Check sheet for the modelled part. Datum: model origin and axes. Units: mm. A direction names the side the tool comes from. Coordinates: 2 decimals unless noted, no trailing zeros. Loops run counter-clockwise (first coordinate to the right, second up) from the corner with the lowest first, then second, coordinate; pieces in that order, holes last.
Autodesk Inventor part; units mm, degrees
ref_plane "Pracovní rovina1" through (0, 0, 0) normal (0, 0, -1) x (-1, 0, 0)
ref_plane "YZ Plane" through (0, 0, 0) normal (1, 0, 0) x (0, 1, 0)
ref_plane "XZ Plane" through (0, 0, 0) normal (0, 1, 0) x (-1, 0, 0)
sketch "Náčrt1" plane through (0, 0, 0) normal (0, 0, 1) x (1, 0, 0)
  line L0 (-97.4, 0) -> (80.4, 0)
  line L1 (0, -76.3) -> (0, 76.3)
  line L2 (-55, 54.5) -> (55, 54.5)
  line L3 (55, 54.5) -> (55, 20.5)
  line L4 (55, 20.5) -> (-55, 20.5)
  line L5 (-55, 20.5) -> (-55, 54.5)
  line L6 (40, -54.5) -> (8, -54.5)
  line L7 (8, -54.5) -> (8, 20.5)
  line L8 (8, 20.5) -> (40, 20.5)
  line L9 (40, 20.5) -> (40, -54.5)
  circle A0 centre (-55, 37.5) radius 17
  point P0 (0, 0)
  point P1 (-55, 20.5)
  point P2 (40, 20.5)
  dimension "d0" = 34
  dimension "d1" = 110
  dimension "d2" = 32
  dimension "d3" = 15
  dimension "d4" = 75
extrude "Vysunutí1" add sketch "Náčrt1" along normal blind 14 contours L7 L4 L9 L0 | L0 L9 L6 L7 | L4 A0 L2 L1 | L1 L2 L3 L4 | A0 L5 | L5 A0
sketch "Náčrt2" plane through (0, 0, 0) normal (0, 0, -1) x (-1, 0, 0)
  line L0 (-55, 54.5) -> (55, 54.5)
  line L1 (-55, 54.5) -> (55, 54.5)
  line L2 (-55, 20.5) -> (-55, 54.5)
  line L3 (-40, 20.5) -> (-55, 20.5)
  line L4 (-40, -54.5) -> (-40, 20.5)
  line L5 (-8, -54.5) -> (-40, -54.5)
  line L6 (-8, 20.5) -> (-8, -54.5)
  line L7 (55, 20.5) -> (-8, 20.5)
  arc A0 (55, 20.5) -> (55, 54.5) centre (55, 37.5) ccw
  point P0 (0, 0)
hole "Díra1" at (-55, 37.5, 0) direction (0, 0, 1) diameter 13 end through all counterbore diameter 22 counterbore depth 8
chamfer "Zkosení1" distance 3 angle 45 8 edges at (0, 54.5, 14) (-72, 37.5, 14) (-23.5, 20.5, 14) (8, -17, 14) (40, -17, 14) (47.5, 20.5, 14) (55, 37.5, 14) (24, -54.5, 14)
sketch "Náčrt3" plane through (0, 0, 14) normal (0, 0, 1) x (1, 0, 0)
  circle A0 centre (-55, 37.5) radius 6.5
  line L0 (-55, 51.5) -> (52, 51.5)
  arc A1 (-55, 51.5) -> (-55, 23.5) centre (-55, 37.5) ccw
  line L1 (11, 23.5) -> (-55, 23.5)
  line L2 (11, -51.5) -> (11, 23.5)
  line L3 (37, -51.5) -> (11, -51.5)
  line L4 (37, 23.5) -> (37, -51.5)
  line L5 (52, 23.5) -> (37, 23.5)
  line L6 (52, 51.5) -> (52, 23.5)
  line L7 (0, 76.3) -> (0, -76.3)
  line L8 (-97.4, 0) -> (80.4, 0)
  point P0 (0, 0)
  point P1 (35, 37.5)
  dimension "d17" = 14
  dimension "d18" = 17
hole "Díra2" at (35, 37.5, 14) direction (0, 0, -1) diameter 6.5 end through all counterbore diameter 11 counterbore depth 4
pattern_linear "Obdélníkové pole1" count 2 spacing 20 along (-1, 0, 0) of "Díra2"
sketch "Náčrt4" plane through (0, 0, 14) normal (0, 0, 1) x (1, 0, 0)
  line L0 (-97.4, 0) -> (80.4, 0)
  line L1 (0, -76.3) -> (0, 76.3)
  circle A0 centre (15, 37.5) radius 5.5
  circle A1 centre (35, 37.5) radius 5.5
  circle A2 centre (-55, 37.5) radius 6.5
  line L2 (-55, 51.5) -> (52, 51.5)
  arc A3 (-55, 51.5) -> (-55, 23.5) centre (-55, 37.5) ccw
  line L3 (11, 23.5) -> (-55, 23.5)
  line L4 (11, -51.5) -> (11, 23.5)
  line L5 (37, -51.5) -> (11, -51.5)
  line L6 (37, 23.5) -> (37, -51.5)
  line L7 (52, 23.5) -> (37, 23.5)
  line L8 (52, 51.5) -> (52, 23.5)
  line L9 (-31.453, 27.5) -> (-26.453, 27.5)
  line L10 (-26.453, 27.5) -> (-38, 47.5)
  line L11 (-26.453, 27.5) -> (-3.359, 27.5) construction
  line L12 (-31.453, 27.5) -> (-43, 47.5)
  line L13 (-43, 47.5) -> (-38, 47.5)
  point P0 (0, 0)
  dimension "d29" = 120
  dimension "d31" = 5
  dimension "d32" = 4
  dimension "d33" = 4
  dimension "d34" = 12
extrude "Vysunutí2" cut sketch "Náčrt4" against normal through all contours L12 L13 L10 L9
chamfer "Zkosení2" distance 1 angle 45 4 edges at (-37.2265, 37.5, 14) (-40.5, 47.5, 14) (-32.2265, 37.5, 14) (-28.953, 27.5, 14)
pattern_linear "Obdélníkové pole2" count 3 spacing 12 along (1, 0, 0) of "Vysunutí2", "Zkosení2"
sketch "Náčrt5" plane through (0, 0, 14) normal (0, 0, 1) x (1, 0, 0)
  line L0 (-32.7321, 48.5) -> (-20.0303, 26.5)
  line L1 (-25.4226, 48.5) -> (-32.7321, 48.5)
  line L2 (-12.7209, 26.5) -> (-25.4226, 48.5)
  line L3 (-20.0303, 26.5) -> (-12.7209, 26.5)
  line L4 (-55, 51.5) -> (52, 51.5)
  arc A0 (-55, 51.5) -> (-55, 23.5) centre (-55, 37.5) ccw
  line L5 (11, 23.5) -> (-55, 23.5)
  line L6 (11, -51.5) -> (11, 23.5)
  line L7 (37, -51.5) -> (11, -51.5)
  line L8 (37, 23.5) -> (37, -51.5)
  line L9 (52, 23.5) -> (37, 23.5)
  line L10 (52, 51.5) -> (52, 23.5)
  circle A1 centre (-55, 37.5) radius 6.5
  circle A2 centre (35, 37.5) radius 5.5
  circle A3 centre (15, 37.5) radius 5.5
  line L11 (-24.7209, 26.5) -> (-37.4226, 48.5)
  line L12 (-32.0303, 26.5) -> (-24.7209, 26.5)
  line L13 (-44.7321, 48.5) -> (-32.0303, 26.5)
  line L14 (-37.4226, 48.5) -> (-44.7321, 48.5)
  line L15 (-20.7321, 48.5) -> (-8.0303, 26.5)
  line L16 (-13.4226, 48.5) -> (-20.7321, 48.5)
  line L17 (-0.7209, 26.5) -> (-13.4226, 48.5)
  line L18 (-8.0303, 26.5) -> (-0.7209, 26.5)
  line L19 (0, -76.3) -> (0, 76.3)
  line L20 (26, 17.9641) -> (28, 14.5)
  line L21 (28, 14.5) -> (26, 11.0359)
  line L22 (26, 11.0359) -> (22, 11.0359)
  line L23 (22, 11.0359) -> (20, 14.5)
  line L24 (20, 14.5) -> (22, 17.9641)
  line L25 (22, 17.9641) -> (26, 17.9641)
  point P0 (0, 0)
  point P1 (24, 14.5)
  dimension "d43" = 4
  dimension "d44" = 9
  dimension "d45" = 13
  dimension "d52" = 3.4641
extrude "Vysunutí3" cut sketch "Náčrt5" against normal through all contours L20 L21 L22 L23 L24 L25
chamfer "Zkosení3" distance 1 angle 45 6 edges at (24, 17.9641, 14) (27, 16.2321, 14) (27, 12.7679, 14) (24, 11.0359, 14) (21, 12.7679, 14) (21, 16.2321, 14)
pattern_linear "Obdélníkové pole3" count 4 spacing 18 along (0, -1, 0) of "Vysunutí3", "Zkosení3"
ref_plane "Pracovní rovina1" through (0, 0, 0) normal (0, 0, -1) x (-1, 0, 0)
sketch "Náčrt7" plane through (0, 0, 0) normal (0, 0, -1) x (-1, 0, 0)
  line L0 (-28, -39.5) -> (-26, -36.0359)
  line L1 (-26, -36.0359) -> (-22, -36.0359)
  line L2 (-22, -36.0359) -> (-20, -39.5)
  line L3 (-20, -39.5) -> (-22, -42.9641)
  line L4 (-22, -42.9641) -> (-26, -42.9641)
  line L5 (-26, -42.9641) -> (-28, -39.5)
  line L6 (-28, -21.5) -> (-26, -18.0359)
  line L7 (-26, -18.0359) -> (-22, -18.0359)
  line L8 (-22, -18.0359) -> (-20, -21.5)
  line L9 (-20, -21.5) -> (-22, -24.9641)
  line L10 (-22, -24.9641) -> (-26, -24.9641)
  line L11 (-26, -24.9641) -> (-28, -21.5)
  line L12 (-28, -3.5) -> (-26, -0.0359)
  line L13 (-26, -0.0359) -> (-22, -0.0359)
  line L14 (-22, -0.0359) -> (-20, -3.5)
  line L15 (-20, -3.5) -> (-22, -6.9641)
  line L16 (-22, -6.9641) -> (-26, -6.9641)
  line L17 (-26, -6.9641) -> (-28, -3.5)
  line L18 (-20, 14.5) -> (-22, 11.0359)
  line L19 (-22, 11.0359) -> (-26, 11.0359)
  line L20 (-26, 11.0359) -> (-28, 14.5)
  line L21 (-28, 14.5) -> (-26, 17.9641)
  line L22 (-26, 17.9641) -> (-22, 17.9641)
  line L23 (-22, 17.9641) -> (-20, 14.5)
  line L24 (19, 47.5) -> (7.453, 27.5)
  line L25 (7.453, 27.5) -> (2.453, 27.5)
  line L26 (2.453, 27.5) -> (14, 47.5)
  line L27 (14, 47.5) -> (19, 47.5)
  line L28 (31, 47.5) -> (19.453, 27.5)
  line L29 (19.453, 27.5) -> (14.453, 27.5)
  line L30 (14.453, 27.5) -> (26, 47.5)
  line L31 (26, 47.5) -> (31, 47.5)
  line L32 (26.453, 27.5) -> (38, 47.5)
  line L33 (38, 47.5) -> (43, 47.5)
  line L34 (43, 47.5) -> (31.453, 27.5)
  line L35 (31.453, 27.5) -> (26.453, 27.5)
  circle A0 centre (-15, 37.5) radius 3.25
  circle A1 centre (-35, 37.5) radius 3.25
  circle A2 centre (55, 37.5) radius 11
  line L36 (-55, 54.5) -> (55, 54.5)
  line L37 (-55, 20.5) -> (-55, 54.5)
  line L38 (-40, 20.5) -> (-55, 20.5)
  line L39 (-40, -54.5) -> (-40, 20.5)
  line L40 (-8, -54.5) -> (-40, -54.5)
  line L41 (-8, 20.5) -> (-8, -54.5)
  line L42 (55, 20.5) -> (-8, 20.5)
  arc A3 (55, 20.5) -> (55, 54.5) centre (55, 37.5) ccw
  line L43 (-40, 11.8397) -> (-55, 20.5)
  line L44 (-8, 11.8397) -> (7, 20.5)
  line L45 (-8, 20.5) -> (-8, -54.5)
  line L46 (-8, 11.8397) -> (-8, 20.5)
  line L47 (-8, 20.5) -> (7, 20.5)
  line L48 (-40, -54.5) -> (-40, 20.5)
  line L49 (-40, 11.8397) -> (-40, 20.5)
  line L50 (-40, 20.5) -> (-55, 20.5)
  point P0 (0, 0)
  dimension "d68" = 15
  dimension "d69" = 15
  dimension "d70" = 30
  dimension "d71" = 30
extrude "Vysunutí4" add sketch "Náčrt7" against normal blind 11 contours L38 L39 L43 | L44 L41 L42
properties part number "blet_leg_30x30 - rozsirene_3D tisk"
1) Section check C-C on y = -32.5. Enter the section's corners in (x, z), plus the area to 3 significant figures.
Answer sheet:
outline: (8, 0) - (40, 0) - (40, 11) - (37, 14) - (11, 14) - (8, 11) - close
area: 439 mm2
2) Section check B-B on z = 6. Give the number of separate pieces and of enclosed holes in the cut face, plus the area to 3 significant figures.
Answer sheet:
separate pieces: 1
enclosed holes: 10
area: 5,810 mm2
3) Section check D-D on x = 1.5. Enter the section's corners in (y, z), plus the area to 3 significant figures.
Answer sheet:
outline: (15.59, 0) - (54.5, 0) - (54.5, 11) - (51.5, 14) - (23.5, 14) - (20.5, 11) - (15.59, 11) - close
area: 521 mm2
4) Depth check by flat-ended pin: pin 1 (7 mm diameter, centred on x = 48, y = 15, fed in from +Z); pin 2 (10.5 mm diameter, centred on x = -55, y = 37.5, fed in from -Z); pin 3 (8 mm diameter, centred on x = -55, z = 10, fed in from -Y); pin 4 (3 mm diameter, centred on y = 30, z = 9.5, fed in from -X). Enter the tip coordinate at first touch or a pass-through.
Answer sheet:
pin 1: stops at z = 11
pin 2: passes through
pin 3: stops at y = 20.5
pin 4: stops at x = -70.91
5) Scan lines: line 1 (X direction, y = -37, z = 1.5); line 2 (Y direction, x = 17, z = 11.25); line 3 (X direction, y = -14.5, z = 1.25). Record each from-to range of solid material in increasing order.
Answer sheet:
line 1: x = 8 to 21.44, 26.56 to 40
line 2: y = -54.25 to 32.38, 42.62 to 54.25
line 3: x = 8 to 40
6) Section check A-A on x = 35. Enter the section's corners in (y, z).
Answer sheet:
outline: (-54.5, 0) - (34.25, 0) - (34.25, 10) - (32, 10) - (32, 14) - (-51.5, 14) - (-54.5, 11) - close; (40.75, 0) - (54.5, 0) - (54.5, 11) - (51.5, 14) - (43, 14) - (43, 10) - (40.75, 10) - close
7) Mould release check, pull along X, two halves, no side actions. Record for faces 1 (the flat face through (21.014, 12.744, 6.591)), 2 (the conical face through (-69.184, 37.188, 13.812)), 3 (the flat face through (-0.8, 53, 12.5)): +X half, -X half, draft (parallel to the pull), parting line (faces both ways), or undercut.
Answer sheet:
face 1: undercut
face 2: -X half
face 3: draft
8) Set-up check for faces 4 (the flat face through (-38.03, 37.91, 13.49)), 5 (the flat face through (2, 17, 11)), 6 (the flat face through (24, -6.964, 7)), 7 (the flat face through (-31, 20.5, 5)): record each of +Z, -Z, +X, -X, +Y, -Y from which the full face is reachable in a straight line by a thin tool's end or side.
Answer sheet:
face 4: +Z
face 5: +Z, -X, -Y
face 6: +Z, -Z
face 7: +Z, -Z, -X, -Y
